For this review, use the dimensioned drawing (mm, ordinates from the lowest corner) and the shaded views. Round coordinates to 2 decimals unless told otherwise and drop trailing zeros. Order: outer loops, then holes, each group sorted by start corner. A loop starts at its lowest first (then second) coordinate and runs counter-clockwise, first axis right, second up. Notation, with made-up numbers: (34, 54.5) - (79, 54.5) arc R28 ccw to (79, 73.5) - close; hole circle Ø1 at (65, 69). An arc over 180 degrees is marked (long way). Write each question's results on one line, items separated by ' | '. Start each with the question number.
(1) For L1, parallel to X at y = 2, z = 175.5; L2, parallel to Z at x = 8, y = 2.85; L3, parallel to Z at x = 56.5, y = 1.55, list the stretches that pass through material, from the lowest coordinate up. Write a range as from..to.
(2) Take a section at B-B, the plane x = 44. Give the boundary of the cut face in (y, z), plus the area to 3 significant figures.
(3) Take a section at A-A, the plane y = 1.4. Give the number of separate pieces and of enclosed holes in the cut face, plus the area to 3 significant figures.
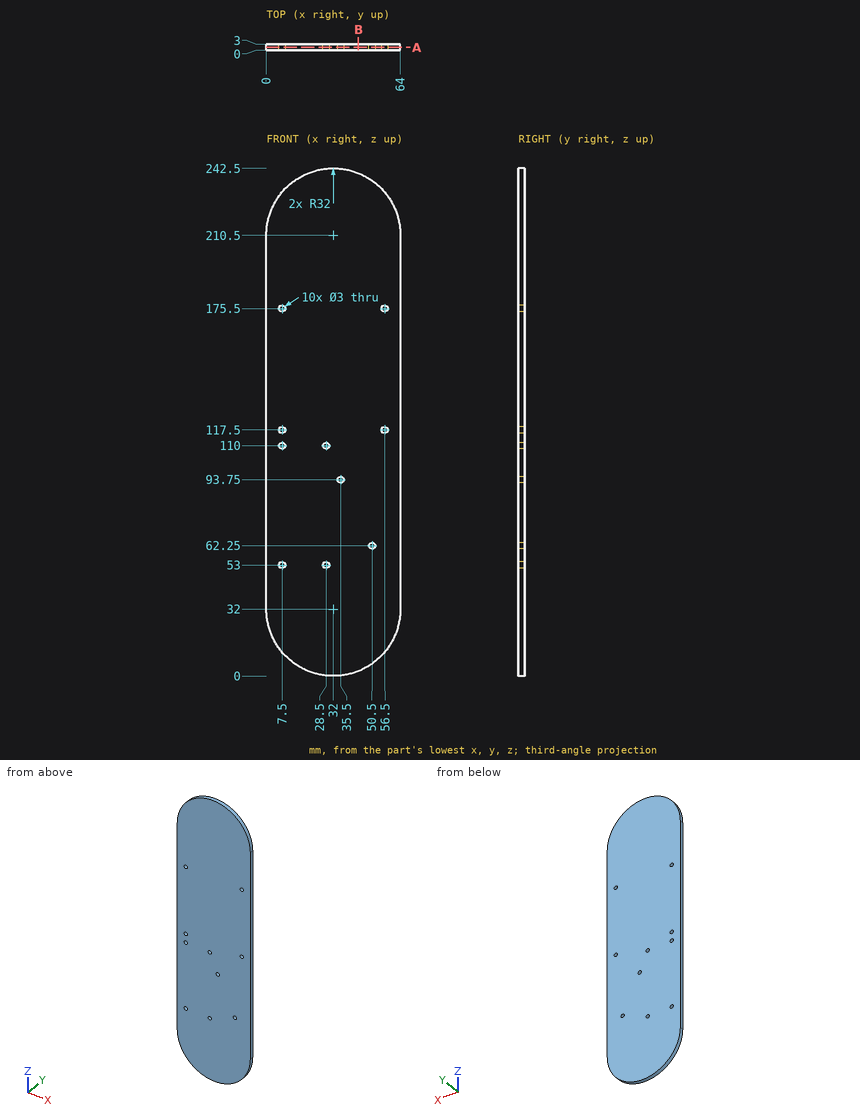
Results below:
1) L1: x = 0..6, 9..55, 58..64 | L2: z = 10.83..51.59, 54.41..108.59, 111.41..116.09, 118.91..174.09, 176.91..231.67 | L3: z = 11.41..116, 119..174, 177..231.09
2) outline: (0, 2.34) - (3, 2.34) - (3, 240.16) - (0, 240.16) - close | area: 713 mm^2
3) separate pieces: 1 | enclosed holes: 10 | area: 14,600 mm^2
